Work out the finished part from the listing and answer in its coordinate system (mm). A direction names the side the tool comes from. Coordinates: 2 decimals unless noted, no trailing zeros. Loops run counter-clockwise (first coordinate to the right, second up) from the corner with the lowest first, then second, coordinate; pieces in that order, holes last. Notation, with made-up numbers: (56, 20) -> (85, 20) arc R29 ccw to (85, 44) -> close; hole circle Ø8 at (78.5, 73). An arc over 180 degrees is marked (long way). One line per question, with ' | ' between items.
```python
from build123d import *

# Parameters (mm, degrees)
F0_W      = 13
F0_H      = 15
F1_DEPTH  = 21
F3_DEPTH  = 21
F4_W      = 5
F4_H      = 15
F5_DEPTH  = 5
F6_R      = 1.75
F7_DEPTH  = 42
F8_R      = 1.75
F9_DEPTH  = 2
F10_R     = 3
F10_R_2   = 1.75
F11_DEPTH = 2
F12_SIZE  = 1.2
F13_R     = 1


# Not quite as in the source:
# - an extrude ends at something that could not be found from the text; its depth is read off the source's solid


with BuildPart() as f1:
    # F0 (on Top) → F1 (new body)
    with BuildSketch(Plane.XY):
        Rectangle(F0_W, F0_H)
    extrude(amount=F1_DEPTH)

    # F2 (on face) → F3 (cut, through all)
    with BuildSketch(Plane.XY.offset(21)):
        with BuildLine():
            ThreePointArc((-0.9255449651, -1.272559936), (-0.682675922, -0.6567701872), (-0.6, 0))
            ThreePointArc((-0.6, 0), (-0.682675922, 0.6567701872), (-0.9255449651, 1.272559936))
            Line((-0.9255449651, 1.272559936), (-0.9255449651, -1.272559936))
        make_face()
        with BuildLine():
            ThreePointArc((-0.9255449651, 1.272559936), (-0.682675922, 0.6567701872), (-0.6, 0))
            ThreePointArc((-0.6, 0), (-0.682675922, -0.6567701872), (-0.9255449651, -1.272559936))
            Line((-0.9255449651, -1.272559936), (6.5, -1.5))
            Line((6.5, -1.5), (6.5, 1.5))
            Line((6.5, 1.5), (-0.9255449651, 1.272559936))
        make_face()
        with BuildLine():
            Line((-0.9255449651, -1.272559936), (-0.9255449651, 1.272559936))
            ThreePointArc((-0.9255449651, 1.272559936), (-5.9, 0), (-0.9255449651, -1.272559936))
        make_face()
    extrude(amount=-F3_DEPTH, mode=Mode.SUBTRACT)

    # F4 (on face) → F5 (cut)
    with BuildSketch(Plane.XY.offset(21)):
        with Locations((4, 0)):
            Rectangle(F4_W, F4_H)
    extrude(amount=-F5_DEPTH, mode=Mode.SUBTRACT)

    # F6 (on face) → F7 (cut, through all)
    with BuildSketch(Plane.XZ.offset(7.5)):
        with Locations((2, 8)):
            Circle(F6_R)
    extrude(amount=-F7_DEPTH, mode=Mode.SUBTRACT)

    # F8 (on face) → F9 (cut)
    with BuildSketch(Plane(origin=(0, 7.5, 0), x_dir=(-1, 0, 0), z_dir=(0, 1, 0))):
        Polygon((-0.2679491924, 11), (-3.7320508076, 11), (-5.4641016151, 8), (-3.7320508076, 5), (-0.2679491924, 5), (1.4641016151, 8), align=None)
        with Locations((-2, 8)):
            Circle(F8_R, mode=Mode.SUBTRACT)
    extrude(amount=-F9_DEPTH, mode=Mode.SUBTRACT)

    # F10 (on face) → F11 (cut)
    with BuildSketch(Plane.XZ.offset(7.5)):
        with Locations((2, 8)):
            Circle(F10_R)
        with Locations((2, 8)):
            Circle(F10_R_2, mode=Mode.SUBTRACT)
    extrude(amount=-F11_DEPTH, mode=Mode.SUBTRACT)

    # F12
    f12_edges = [f1.edges().sort_by_distance(p)[0] for p in [
        (-1, -5.5, 8),
    ]]
    chamfer(f12_edges, length=F12_SIZE)

    # F13
    f13_edges = [f1.edges().sort_by_distance(p)[0] for p in [
        (6.5, -7.5, 8),
        (6.5, 7.5, 8),
    ]]
    fillet(f13_edges, radius=F13_R)


solid = f1.part
```
1) Find section D-D (x = -3.25). Write down the section's boundary in (y, z), plus the area to 3 significant figures.
Check values:
outline: (-7.5, 0) -> (-2.65, 0) -> (-2.65, 21) -> (-7.5, 21) -> close; (2.65, 0) -> (7.5, 0) -> (7.5, 21) -> (2.65, 21) -> close | area: 204 mm^2
2) Find the intervals of material crossed by line 1 along X through (y, z) = (-3.85, 8); line 2 along Z through (x, y) = (1.25, 6); line 3 along Z through (x, y) = (1.75, 5.75), in increasing order.
Check values:
line 1: x = -6.5 to 0.25, 3.75 to 6.5 | line 2: z = 0 to 5, 11 to 21 | line 3: z = 0 to 5, 11 to 16
3) Flat-ended cylindrical pins translate along their axes: pin 1 (2 mm diameter, centred on x = 2, z = 8, fed in from -Y); pin 2 (4.5 mm diameter, centred on x = 2, z = 8, fed in from +Y); pin 3 (2.5 mm diameter, centred on x = 4.5, y = 4, fed in from +Z); pin 4 (1.5 mm diameter, centred on y = 3.5, z = 18, fed in from +X). Find the tip coordinate at first contact, or state that the pin passes through.
Check values:
pin 1: passes through | pin 2: stops at y = 5.5 | pin 3: stops at z = 16 | pin 4: stops at x = 1.5
4) For faces 1 (the face through (4, -4, 16)), 2 (the face through (0, 2, 0)), 3 (the face through (2, 7, 5)), 4 (the face through (3.61, -7.11, 10.53)), determine the directions among +Z, -Z, +X, -X, +Y, -Y from which every point of the face is accessible in a straight line to the end or side of a thin tool.
Check values:
face 1: +Z, +X, +Y, -Y | face 2: -Z, +X, -X, +Y, -Y | face 3: +Y | face 4: -Y
5) Find section C-C (y = 1.75). Write down the section's boundary in (x, z), plus the area to 3 significant figures.
Check values:
outline: (-6.5, 0) -> (-5.24, 0) -> (-5.24, 21) -> (-6.5, 21) -> close; (-1.26, 0) -> (6.5, 0) -> (6.5, 16) -> (1.5, 16) -> (1.5, 21) -> (-1.26, 21) -> close; hole circle Ø3.5 at (2, 8) | area: 155 mm^2
6) Find section A-A (x = 2). Write down the section's boundary in (y, z).
Check values:
outline: (-7.5, 0) -> (-1.36, 0) -> (-1.36, 6.25) -> (-5.5, 6.25) -> (-5.5, 6.2) -> (-6.7, 5) -> (-7.5, 5) -> close; (-7.5, 11) -> (-6.7, 11) -> (-5.5, 9.8) -> (-5.5, 9.75) -> (-1.36, 9.75) -> (-1.36, 16) -> (-7.5, 16) -> close; (1.36, 0) -> (7.5, 0) -> (7.5, 5) -> (5.5, 5) -> (5.5, 6.25) -> (1.36, 6.25) -> close; (1.36, 9.75) -> (5.5, 9.75) -> (5.5, 11) -> (7.5, 11) -> (7.5, 16) -> (1.36, 16) -> close
7) Find section B-B (z = 19.5). Write down the section's boundary in (x, y).
Check values:
outline: (-6.5, -7.5) -> (1.5, -7.5) -> (1.5, -1.35) -> (-0.93, -1.27) arc R2.65 cw (long way) to (-0.93, 1.27) -> (1.5, 1.35) -> (1.5, 7.5) -> (-6.5, 7.5) -> close
